```python
from build123d import *

# Parameters (mm, degrees)
SKETCH_1_R      = 2.55
SKETCH_1_R_2    = 6
EXTRUDE_1_DEPTH = 9
FILLET_1_R      = 5


with BuildPart() as part:
    # 草图1 → 凸台-拉伸1 (new body)
    with BuildSketch(Plane.XY):
        Polygon((-54.053450796, 27.320514858), (5.802955665, 27.320514858), (-28.018037849, -17.774143161), align=None)
        with Locations((-40.197044335, 19.320514858)):
            Circle(SKETCH_1_R, mode=Mode.SUBTRACT)
        with Locations((-27.148108815, -3.280904448)):
            Circle(SKETCH_1_R, mode=Mode.SUBTRACT)
        with Locations((-10.197044335, 19.320514858)):
            Circle(SKETCH_1_R, mode=Mode.SUBTRACT)
        with Locations((-24.197044335, 12.320514858)):
            Circle(SKETCH_1_R_2, mode=Mode.SUBTRACT)
    extrude(amount=EXTRUDE_1_DEPTH)

    # 圆角1
    fillet_1_edges = [part.edges().sort_by_distance(p)[0] for p in [
        (-54.053450796, 27.320514858, 4.5),
        (5.802955665, 27.320514858, 4.5),
        (-28.018037849, -17.774143161, 4.5),
    ]]
    fillet(fillet_1_edges, radius=FILLET_1_R)


solid = part.part
```
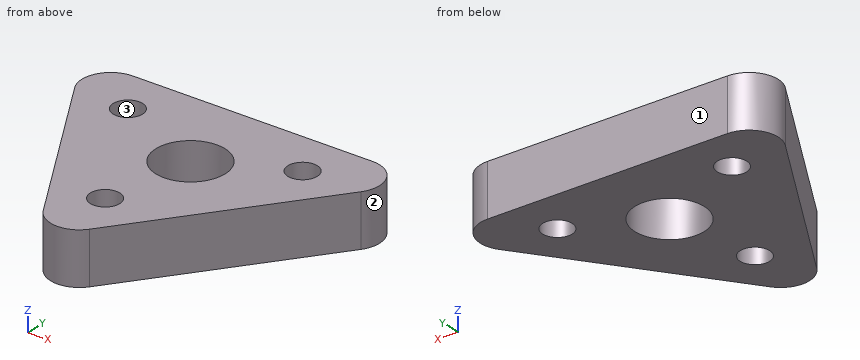
Read the model definition and answer for the solid it produces. Units are mm, in the model's axes. Face numbers are marked on the shaded views. Round coordinates to 2 decimals unless told otherwise and drop trailing zeros. Write each loop counter-clockwise with the first axis right and the second up, starting at its lowest first coordinate (ties: lowest second). Pieces come first, ordered by that corner, then holes. Notation, with made-up numbers: (73.5, 81.25) -> (119.5, 81.25) arc R21 cw to (119.5, 99.25) -> close; hole circle Ø1 at (45.25, 3). An arc over 180 degrees is marked (long way). Answer in a Markdown table with one row per item. Add a question column.
1) Consider line 1 (X direction, y = 19, z = 5); line 2 (X direction, y = 20.5, z = 7.5); line 3 (Y direction, x = -27, z = 7.25). Determine where each line is inside the solid, lowest interval first.
2) Find section D-D, the plane y = 25. Determine the outline of the cut face in (x, z), and give its area (3 significant figures).
3) Find section B-B, the plane x = -39.5. Determine the outline of the cut face in (y, z).
4) Find section A-A, the plane x = -27. Determine the outline of the cut face in (y, z).
5) Determine the mould class of the marked faces 1, 2 and 3 for opening direction Y: pulls with the +Y half, pulls with the -Y half, needs draft (parallel to the pull), parting line crosses it, or undercut.
6) Find section C-C, the plane z = 5. Determine the outline of the cut face in (x, y).
7) Given P1, Ø11, axis at x = -24.2, y = 12.32, coming from the +Z side; P2, Ø2, axis at x = -29, z = 2, coming from the -Y side; P3, Ø1, axis at y = -1, z = 3, coming from the -X side; P4, Ø1, axis at y = 11.5, z = 4.5, coming from the +X side, each flat-ended and moving along its own axis, determine where each tip first touches the part or whether it passes through.
Findings below:
| question | item | result |
|---|---|---|
| 1 | line 1 | -49.25 to -42.73, -37.67 to -12.73, -7.67 to -0.44 |
| 1 | line 2 | -50.05 to -42.46, -37.94 to -12.46, -7.94 to 0.46 |
| 1 | line 3 | -13.69 to -5.83, -0.74 to 7.02, 17.63 to 27.32 |
| 2 | outline | (-49.61, 0) -> (0.02, 0) -> (0.02, 9) -> (-49.61, 9) -> close |
| 2 | area | 447 mm² |
| 3 | outline | (2.11, 0) -> (16.87, 0) -> (16.87, 9) -> (2.11, 9) -> close; (21.77, 0) -> (27.32, 0) -> (27.32, 9) -> (21.77, 9) -> close |
| 4 | outline | (-13.69, 0) -> (-5.83, 0) -> (-5.83, 9) -> (-13.69, 9) -> close; (-0.74, 0) -> (7.02, 0) -> (7.02, 9) -> (-0.74, 9) -> close; (17.63, 0) -> (27.32, 0) -> (27.32, 9) -> (17.63, 9) -> close |
| 5 | face 1 | pulls with the +Y half |
| 5 | face 2 | parting line crosses it |
| 5 | face 3 | undercut |
| 6 | outline | (-49.72, 19.82) -> (-31.8, -11.22) arc R5 ccw to (-23.47, -11.72) -> (-0.2, 19.32) arc R5 ccw to (-4.2, 27.32) -> (-45.39, 27.32) arc R5 ccw to start; hole circle Ø5.1 at (-40.2, 19.32); hole circle Ø12 at (-24.2, 12.32); hole circle Ø5.1 at (-27.15, -3.28); hole circle Ø5.1 at (-10.2, 19.32) |
| 7 | P1 | through |
| 7 | P2 | y = -13.69 |
| 7 | P3 | x = -37.99 |
| 7 | P4 | x = -5.69 |
